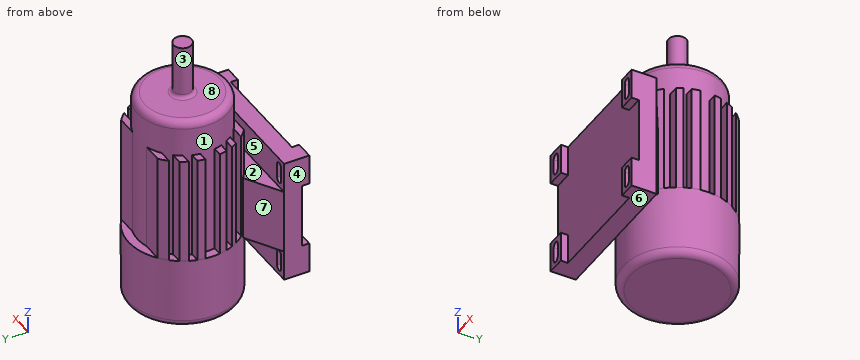
```python
from build123d import *
from build123d.topology import SkipClean

# Parameters (mm, degrees)
SKETCH1_R            = 150
BOSS_EXTRUDE1_DEPTH  = 200
BOSS_EXTRUDE11_DEPTH = 300
BOSS_EXTRUDE14_START = -300
SKETCH12_R           = 125
BOSS_EXTRUDE14_DEPTH = 400
SKETCH13_W           = 46.677917496
SKETCH13_H           = 84.453402707
SKETCH13_H_2         = 84.453402706
SKETCH13_W_2         = 50
BOSS_EXTRUDE15_DEPTH = 50
SKETCH13_3_W         = 46.677917496
SKETCH13_3_H         = 84.453402706
SKETCH13_3_H_2       = 84.453402707
SKETCH13_3_W_2       = 50
BOSS_EXTRUDE16_DEPTH = 20
BOSS_EXTRUDE17_DEPTH = 90
SKETCH16_R           = 25
BOSS_EXTRUDE18_DEPTH = 150
FILLET2_R            = 10
FILLET3_R            = 20


with BuildPart() as part:
    # Sketch1 → Boss-Extrude1 (new body)
    with BuildSketch(Plane.XY):
        Circle(SKETCH1_R)
    extrude(amount=BOSS_EXTRUDE1_DEPTH)

    # Sketch7 → Boss-Extrude11 (add)
    with SkipClean():  # the faces are left unmerged after this step: merging them gives an invalid solid
        with BuildSketch(Plane.XY.offset(200)):
            with BuildLine():
                Line((-90, 120), (90, 120))
                ThreePointArc((90, 120), (101.396020382, 110.538893837), (111.803398875, 100))
                Line((111.803398875, 100), (-111.803398875, 100))
                ThreePointArc((-111.803398875, 100), (-101.396020382, 110.538893837), (-90, 120))
            make_face()
            with BuildLine():
                Line((-126.885775404, 80), (126.885775404, 80))
                ThreePointArc((126.885775404, 80), (132.559251115, 70.200035213), (137.477270849, 60))
                Line((137.477270849, 60), (-137.477270849, 60))
                ThreePointArc((-137.477270849, 60), (-132.559251115, 70.200035213), (-126.885775404, 80))
            make_face()
            with BuildLine():
                Line((144.16342013, -41.435592144), (-144.16342013, -41.435592144))
                ThreePointArc((-144.16342013, -41.435592144), (-146.803816882, -30.799989431), (-148.660687473, -20))
                Line((-148.660687473, -20), (148.660687473, -20))
                ThreePointArc((148.660687473, -20), (146.803816882, -30.799989431), (144.16342013, -41.435592144))
            make_face()
            with BuildLine():
                Line((111.803398875, -100), (-111.803398875, -100))
                ThreePointArc((-111.803398875, -100), (-101.396020382, -110.538893837), (-90, -120))
                Line((-90, -120), (90, -120))
                ThreePointArc((90, -120), (101.396020382, -110.538893837), (111.803398875, -100))
            make_face()
            with BuildLine():
                Line((144.568322948, 40), (-144.568322948, 40))
                ThreePointArc((-144.568322948, 40), (-146.955139883, 30.069700063), (-148.660687473, 20))
                Line((-148.660687473, 20), (148.660687473, 20))
                ThreePointArc((148.660687473, 20), (146.955139883, 30.069700063), (144.568322948, 40))
            make_face()
            with BuildLine():
                Line((137.477270849, -60), (-137.477270849, -60))
                ThreePointArc((-137.477270849, -60), (-133.599215205, -68.20007109), (-129.232599216, -76.150740639))
                Line((-129.232599216, -76.150740639), (129.232599216, -76.150740639))
                ThreePointArc((129.232599216, -76.150740639), (133.599215205, -68.20007109), (137.477270849, -60))
            make_face()
        extrude(amount=BOSS_EXTRUDE11_DEPTH)



with BuildPart() as body_2:
    # Sketch12 → Boss-Extrude14 (new body)
    with BuildSketch(Plane.XY.offset(500).offset(BOSS_EXTRUDE14_START)):
        Circle(SKETCH12_R)
    extrude(amount=BOSS_EXTRUDE14_DEPTH)


with BuildPart() as body_3:
    # Sketch13 → Boss-Extrude15 (new body)
    # profile 1 of 5: a face of its own
    with BuildSketch(Plane(origin=(0, -220, 0), x_dir=(-1, 0, 0), z_dir=(0, -1, 0))):
        Polygon((150, -99.735715433), (-153.322082504, -99.735715433), (-153.322082504, -184.18911814), (-200, -184.18911814), (-200, -365.282312727), (-153.322082504, -365.282312727), (-153.322082504, -449.735715433), (150, -449.735715433), (150, -365.282312727), (200, -365.282312727), (200, -184.18911814), (150, -184.18911814), align=None)
    # profile 2 of 5: a face of its own
    with BuildSketch(Plane(origin=(0, -220, 0), x_dir=(-1, 0, 0), z_dir=(0, -1, 0))):
        with Locations((-176.661041252, -141.962416787)):
            Rectangle(SKETCH13_W, SKETCH13_H)
        with BuildLine():
            ThreePointArc((-186.661041252, -121.962416787), (-176.661041252, -111.962416787), (-166.661041252, -121.962416787))
            Line((-166.661041252, -121.962416787), (-166.661041252, -161.962416787))
            ThreePointArc((-166.661041252, -161.962416787), (-176.661041252, -171.962416787), (-186.661041252, -161.962416787))
            Line((-186.661041252, -161.962416787), (-186.661041252, -121.962416787))
        make_face(mode=Mode.SUBTRACT)
    # profile 3 of 5: a face of its own
    with BuildSketch(Plane(origin=(0, -220, 0), x_dir=(-1, 0, 0), z_dir=(0, -1, 0))):
        with Locations((-176.661041252, -407.50901408)):
            Rectangle(SKETCH13_W, SKETCH13_H_2)
        with BuildLine():
            Line((-166.661041252, -387.50901408), (-166.661041252, -427.50901408))
            ThreePointArc((-166.661041252, -427.50901408), (-176.661041252, -437.50901408), (-186.661041252, -427.50901408))
            Line((-186.661041252, -427.50901408), (-186.661041252, -387.50901408))
            ThreePointArc((-186.661041252, -387.50901408), (-176.661041252, -377.50901408), (-166.661041252, -387.50901408))
        make_face(mode=Mode.SUBTRACT)
    # profile 4 of 5: a face of its own
    with BuildSketch(Plane(origin=(0, -220, 0), x_dir=(-1, 0, 0), z_dir=(0, -1, 0))):
        with Locations((175, -407.50901408)):
            Rectangle(SKETCH13_W_2, SKETCH13_H_2)
        with BuildLine():
            Line((185, -387.50901408), (185, -427.50901408))
            ThreePointArc((185, -427.50901408), (175, -437.50901408), (165, -427.50901408))
            Line((165, -427.50901408), (165, -387.50901408))
            ThreePointArc((165, -387.50901408), (175, -377.50901408), (185, -387.50901408))
        make_face(mode=Mode.SUBTRACT)
    # profile 5 of 5: a face of its own
    with BuildSketch(Plane(origin=(0, -220, 0), x_dir=(-1, 0, 0), z_dir=(0, -1, 0))):
        with Locations((175, -141.962416787)):
            Rectangle(SKETCH13_W_2, SKETCH13_H)
        with BuildLine():
            ThreePointArc((165, -121.962416787), (175, -111.962416787), (185, -121.962416787))
            Line((185, -121.962416787), (185, -161.962416787))
            ThreePointArc((185, -161.962416787), (175, -171.962416787), (165, -161.962416787))
            Line((165, -161.962416787), (165, -121.962416787))
        make_face(mode=Mode.SUBTRACT)
    extrude(amount=-BOSS_EXTRUDE15_DEPTH)

    # Sketch13<3> → Boss-Extrude16 (add)
    # profile 1 of 4: a face of its own
    with BuildSketch(Plane(origin=(0, -220, 0), x_dir=(-1, 0, 0), z_dir=(0, -1, 0))):
        with Locations((-176.661041252, -407.50901408)):
            Rectangle(SKETCH13_3_W, SKETCH13_3_H)
        with BuildLine():
            Line((-166.661041252, -387.50901408), (-166.661041252, -427.50901408))
            ThreePointArc((-166.661041252, -427.50901408), (-176.661041252, -437.50901408), (-186.661041252, -427.50901408))
            Line((-186.661041252, -427.50901408), (-186.661041252, -387.50901408))
            ThreePointArc((-186.661041252, -387.50901408), (-176.661041252, -377.50901408), (-166.661041252, -387.50901408))
        make_face(mode=Mode.SUBTRACT)
    # profile 2 of 4: a face of its own
    with BuildSketch(Plane(origin=(0, -220, 0), x_dir=(-1, 0, 0), z_dir=(0, -1, 0))):
        with Locations((-176.661041252, -141.962416787)):
            Rectangle(SKETCH13_3_W, SKETCH13_3_H_2)
        with BuildLine():
            ThreePointArc((-186.661041252, -121.962416787), (-176.661041252, -111.962416787), (-166.661041252, -121.962416787))
            Line((-166.661041252, -121.962416787), (-166.661041252, -161.962416787))
            ThreePointArc((-166.661041252, -161.962416787), (-176.661041252, -171.962416787), (-186.661041252, -161.962416787))
            Line((-186.661041252, -161.962416787), (-186.661041252, -121.962416787))
        make_face(mode=Mode.SUBTRACT)
    # profile 3 of 4: a face of its own
    with BuildSketch(Plane(origin=(0, -220, 0), x_dir=(-1, 0, 0), z_dir=(0, -1, 0))):
        with Locations((175, -407.50901408)):
            Rectangle(SKETCH13_3_W_2, SKETCH13_3_H)
        with BuildLine():
            Line((185, -387.50901408), (185, -427.50901408))
            ThreePointArc((185, -427.50901408), (175, -437.50901408), (165, -427.50901408))
            Line((165, -427.50901408), (165, -387.50901408))
            ThreePointArc((165, -387.50901408), (175, -377.50901408), (185, -387.50901408))
        make_face(mode=Mode.SUBTRACT)
    # profile 4 of 4: a face of its own
    with BuildSketch(Plane(origin=(0, -220, 0), x_dir=(-1, 0, 0), z_dir=(0, -1, 0))):
        with Locations((175, -141.962416787)):
            Rectangle(SKETCH13_3_W_2, SKETCH13_3_H_2)
        with BuildLine():
            ThreePointArc((165, -121.962416787), (175, -111.962416787), (185, -121.962416787))
            Line((185, -121.962416787), (185, -161.962416787))
            ThreePointArc((185, -161.962416787), (175, -171.962416787), (165, -161.962416787))
            Line((165, -161.962416787), (165, -121.962416787))
        make_face(mode=Mode.SUBTRACT)
    extrude(amount=BOSS_EXTRUDE16_DEPTH)


with BuildPart() as part_1:
    with SkipClean():  # the faces are left unmerged after this step: merging them gives an invalid solid
        add(part.part)

        add(body_2.part)  # Boss-Extrude17 merges body 2

        add(body_3.part)  # Boss-Extrude17 merges body 3
        # Sketch14 → Boss-Extrude17 (add, symmetric)
        with BuildSketch(Plane.XY.offset(274.735715433)):
            Polygon((-200, -170), (200, -170), (100, -110), (-100, -110), align=None)
        extrude(amount=BOSS_EXTRUDE17_DEPTH, both=True)

    # Sketch16 → Boss-Extrude18 (add)
    with BuildSketch(Plane.XY.offset(600)):
        Circle(SKETCH16_R)
    extrude(amount=BOSS_EXTRUDE18_DEPTH)

    # Fillet2
    fillet2_edges = [part_1.edges().sort_by_distance(p)[0] for p in [
        (-25, 0, 600),
    ]]
    fillet(fillet2_edges, radius=FILLET2_R)

    # Fillet3
    fillet3_edges = [part_1.edges().sort_by_distance(p)[0] for p in [
        (-125, 0, 600),
        (-150, 0, 0),
    ]]
    fillet(fillet3_edges, radius=FILLET3_R)


solid = part_1.part
```
Check sheet for the modelled part. Datum: model origin and axes. Units: mm. Face numbers are marked on the shaded views. A direction names the side the tool comes from. Round coordinates to 2 decimals unless told otherwise and drop trailing zeros. Loops run counter-clockwise (first coordinate to the right, second up) from the corner with the lowest first, then second, coordinate; pieces in that order, holes last. Notation, with made-up numbers: (-18, 71) -> (24, 71) arc R27 cw to (24, 91) -> close; hole circle Ø7 at (42, 23). An arc over 180 degrees is marked (long way). Write item = value, one per line. Start each with the question number.
1) Gauge pin test, flat ends, axial feed: pin 1 Ø8.5 at (x, z) = (-126, 383.5) entering from -Y; pin 2 Ø5 at (x, z) = (19.5, 604) entering from -Y; pin 3 Ø5 at (x, z) = (92, 548.5) entering from +Y. Record the tip position at first contact, or that the pin passes through.
2) Sectioned sample at A-A, the plane x = -175. Record the cut outline in (y, z).
3) Sectioned sample at B-B, the plane y = 0. Record the cut outline in (x, z).
4) Release check for a two-part mould opening along Y. For the marked faces 1, 2, 3 and 4 record: released by +Y, released by -Y, zero draft, split by the parting line, or undercut.
5) Set-up check for the marked faces 5, 6, 7 and 8: record each of +Z, -Z, +X, -X, +Y, -Y from which the full face is reachable in a straight line by a thin tool's end or side.
6) Sectioned sample at C-C, the plane x = 0. Record the cut outline in (y, z), plus the area to 3 significant figures.
7) Thickness scan on probe 1 along Y at (x, z) = (-102, 264.5); probe 2 along Y at (x, z) = (62, 449); probe 3 along Z at (x, y) = (-18, -42.5). Record the ranges inside material, lowest first.
Results are:
q1.pin_1 = -220
q1.pin_2 = -22.86
q1.pin_3 = 87.26
q2.outline = (-240, 99.74) -> (-170, 99.74) -> (-170, 111.96) -> (-240, 111.96) -> close; (-240, 171.96) -> (-170, 171.96) -> (-170, 184.74) -> (-155, 184.74) -> (-155, 364.74) -> (-170, 364.74) -> (-170, 377.51) -> (-240, 377.51) -> (-240, 365.28) -> (-220, 365.28) -> (-220, 184.19) -> (-240, 184.19) -> close; (-240, 437.51) -> (-170, 437.51) -> (-170, 449.74) -> (-240, 449.74) -> close
q3.outline = (-150, 20) arc R20 ccw to (-130, 0) -> (130, 0) arc R20 ccw to (150, 20) -> (150, 200) -> (125, 200) -> (125, 580) arc R20 ccw to (105, 600) -> (35, 600) arc R10 cw to (25, 610) -> (25, 750) -> (-25, 750) -> (-25, 610) arc R10 cw to (-35, 600) -> (-105, 600) arc R20 ccw to (-125, 580) -> (-125, 200) -> (-150, 200) -> close
q4.face_1 = undercut
q4.face_2 = undercut
q4.face_3 = split by the parting line
q4.face_4 = zero draft
q5.face_5 = +Z, +X, -X
q5.face_6 = -Z, +X, -X, -Y
q5.face_7 = +Z, -Z, -X
q5.face_8 = +Z
q6.outline = (-220, 99.74) -> (-170, 99.74) -> (-170, 184.74) -> (-150, 184.74) -> (-150, 20) arc R20 ccw to (-130, 0) -> (130, 0) arc R20 ccw to (150, 20) -> (150, 200) -> (125, 200) -> (125, 580) arc R20 ccw to (105, 600) -> (35, 600) arc R10 cw to (25, 610) -> (25, 750) -> (-25, 750) -> (-25, 610) arc R10 cw to (-35, 600) -> (-105, 600) arc R20 ccw to (-125, 580) -> (-125, 364.74) -> (-170, 364.74) -> (-170, 449.74) -> (-220, 449.74) -> close
q6.area = 192,000 mm^2
q7.probe_1 = -220 to -111.2, -109.98 to -100, -76.15 to 80, 100 to 109.98
q7.probe_2 = -220 to -170, -120 to 120
q7.probe_3 = 0 to 600
